```python
from build123d import *

# Parameters (mm, degrees)
SKETCH_1_W          = 60
SKETCH_1_H          = 110
SKETCH_1_R          = 14
SKETCH_1_R_2        = 2
SKETCH_1_R_3        = 2.1
SKETCH_1_R_4        = 1.55
EXTRUDE_1_DEPTH     = 2
CHAMFER_1_SIZE      = 10
CUT_EXTRUDE_1_DEPTH = 63.777384463


with BuildPart() as part:
    # 草图1 → 凸台-拉伸1 (new, symmetric)
    with BuildSketch(Plane.XY):
        Rectangle(SKETCH_1_W, SKETCH_1_H)
        Circle(SKETCH_1_R, mode=Mode.SUBTRACT)
        with Locations((-20, 45)):
            Circle(SKETCH_1_R_2, mode=Mode.SUBTRACT)
        with Locations((20, 45)):
            Circle(SKETCH_1_R_3, mode=Mode.SUBTRACT)
        with Locations((-20, -45)):
            Circle(SKETCH_1_R_2, mode=Mode.SUBTRACT)
        with Locations((20, -45)):
            Circle(SKETCH_1_R_3, mode=Mode.SUBTRACT)
        with Locations((0, 17.5)):
            Circle(SKETCH_1_R_4, mode=Mode.SUBTRACT)
        with Locations((12.374368671, 12.374368671)):
            Circle(SKETCH_1_R_4, mode=Mode.SUBTRACT)
        with Locations((17.5, 0)):
            Circle(SKETCH_1_R_4, mode=Mode.SUBTRACT)
        with Locations((12.374368671, -12.374368671)):
            Circle(SKETCH_1_R_4, mode=Mode.SUBTRACT)
        with Locations((0, -17.5)):
            Circle(SKETCH_1_R_4, mode=Mode.SUBTRACT)
        with Locations((-12.374368671, -12.374368671)):
            Circle(SKETCH_1_R_4, mode=Mode.SUBTRACT)
        with Locations((-17.5, 0)):
            Circle(SKETCH_1_R_4, mode=Mode.SUBTRACT)
        with Locations((-12.374368671, 12.374368671)):
            Circle(SKETCH_1_R_4, mode=Mode.SUBTRACT)
    extrude(amount=EXTRUDE_1_DEPTH, both=True)

    # 倒角1
    chamfer_1_edges = [part.edges().sort_by_distance(p)[0] for p in [
        (-30, 55, 0),
        (30, 55, 0),
        (30, -55, 0),
        (-30, -55, 0),
    ]]
    chamfer(chamfer_1_edges, length=CHAMFER_1_SIZE)

    # 草图2 → 切除-拉伸1 (cut, through all)
    with BuildSketch(Plane(origin=(0, 0, -2), x_dir=(-1, 0, 0), z_dir=(0, 0, -1))):
        Polygon((-30, -10), (-27, -7.5), (-27, 7.5), (-30, 10), align=None)
    extrude(amount=-CUT_EXTRUDE_1_DEPTH, mode=Mode.SUBTRACT)


solid = part.part
```
Build history of the part. All positions in model axes, mm. A direction names the side the tool comes from. Round coordinates to 2 decimals unless told otherwise and drop trailing zeros. Write each loop counter-clockwise with the first axis right and the second up, starting at its lowest first coordinate (ties: lowest second). Pieces come first, ordered by that corner, then holes. Notation, with made-up numbers: (7.5, 67) - (20.5, 67) arc R33 cw to (20.5, 106) - close; hole circle Ø4 at (62.5, -35.75). An arc over 180 degrees is marked (long way). Answer as CSV lines item,"result".
Q1. Pull direction Y, two halves, no side cores. Call faces 1 (the flat face through (25, -50, 0)), 2 (the cylindrical face through (-12.58, 13.91, -0.03)), 3 (the flat face through (-25, 50, 0)): +Y half, -Y half, draft (parallel to the pull), parting line (faces both ways), or undercut.
Report:
face 1,"-Y half"
face 2,"undercut"
face 3,"+Y half"
Q2. Cut at D-D (z = -1.05). State how many separate pieces and enclosed holes the cut face has, and give its area (3 significant figures).
Report:
separate pieces,"1"
enclosed holes,"13"
area,"5,620 mm^2"
Q3. Tool access for faces 4 (the flat face through (28.521, -8.768, -0.028)), 5 (the cylindrical face through (13.853, -11.909, -0.028)): list every direction of +Z, -Z, +X, -X, +Y, -Y with a clear straight run to the whole face (end or side of a thin tool).
Report:
face 4,"+Z, -Z, +X"
face 5,"+Z, -Z"
Q4. Drop flat-ended pins along their axis: pin 1 (1 mm diameter, centred on x = -21.5, z = -0.5, fed in from -Y); pin 2 (2 mm diameter, centred on y = 3.5, z = 0, fed in from +X). Give the stop position or say it passes through.
Report:
pin 1,"stops at y = -54"
pin 2,"stops at x = 27"
Q5. Cut at C-C (x = 4.5). Write the cut outline in (y, z).
Report:
outline,"(-55, -2) - (-13.26, -2) - (-13.26, 2) - (-55, 2) - close; (13.26, -2) - (55, -2) - (55, 2) - (13.26, 2) - close"
Q6. Drill centre lines: probe 1 along Y at (x, z) = (-20, -1); probe 2 along Y at (x, z) = (1, 0.25); probe 3 along X at (y, z) = (-8.5, 0.9). Where is each one in solid material? Low to high. Write a range as [from, to].
Report:
probe 1,"y = [-55, -47], [-43, 43], [47, 55]"
probe 2,"y = [-55, -18.68], [-16.32, -13.96], [13.96, 16.32], [18.68, 55]"
probe 3,"x = [-30, -11.12], [11.12, 28.2]"
Q7. Cut at B-B (y = -17.5). Write the cut outline in (x, z), and give its area (3 significant figures).
Report:
outline,"(-30, -2) - (-1.55, -2) - (-1.55, 2) - (-30, 2) - close; (1.55, -2) - (30, -2) - (30, 2) - (1.55, 2) - close"
area,"228 mm^2"
Q8. Cut at A-A (y = 0). Write the cut outline in (x, z), and give its area (3 significant figures).
Report:
outline,"(-30, -2) - (-19.05, -2) - (-19.05, 2) - (-30, 2) - close; (-15.95, -2) - (-14, -2) - (-14, 2) - (-15.95, 2) - close; (14, -2) - (15.95, -2) - (15.95, 2) - (14, 2) - close; (19.05, -2) - (27, -2) - (27, 2) - (19.05, 2) - close"
area,"91.2 mm^2"
